For this review, take the finished solid that the model builds, in its own axes (mm). Face numbers are marked on the shaded views. A direction names the side the tool comes from. Coordinates: 2 decimals unless noted, no trailing zeros. Loops run counter-clockwise (first coordinate to the right, second up) from the corner with the lowest first, then second, coordinate; pieces in that order, holes last.
Autodesk Inventor part; units mm, degrees
ref_plane "YZ Plane" through (0, 0, 0) normal (1, 0, 0) x (0, 1, 0)
ref_plane "XZ Plane" through (0, 0, 0) normal (0, 1, 0) x (-1, 0, 0)
ref_plane "XY Plane" through (0, 0, 0) normal (0, 0, 1) x (1, 0, 0)
sketch "Sketch1" plane through (0, 0, 0) normal (0, 1, 0) x (-1, 0, 0)
  line L0 (4, -2.4997) -> (79.711, -2.4997)
  line L1 (4, -103.4997) -> (4, -2.4997)
  line L2 (45, -103.4997) -> (4, -103.4997)
  line L3 (69.7122, -36.1325) -> (54.8327, -76.055)
  line L4 (54.8327, -76.055) -> (53.637, -79.4997)
  line L5 (53.637, -79.4997) -> (47.0364, -98.0359)
  line L6 (47.0364, -98.0359) -> (45, -103.4997)
  line L7 (79.711, -2.4997) -> (69.7122, -36.1325)
  line L8 (84.9819, 0) -> (0, 0)
  line L9 (75.6001, -30.2846) -> (84.9819, 0)
  line L10 (84.9819, 0) -> (75.6001, -30.2846)
  line L11 (70.9666, -42.7177) -> (65.5988, -57.1214)
  line L12 (61.2006, -68.9229) -> (56.067, -83.7178)
  line L13 (75.6001, -30.2846) -> (61.2006, -68.9229)
  line L14 (47.8016, -104.8767) -> (46.0595, -108.2232)
  line L15 (50.5948, -98.4014) -> (47.8016, -104.8767)
  line L16 (56.067, -83.7178) -> (50.5948, -98.4014)
  line L17 (0, -108.2232) -> (0, 0)
  line L18 (46.0595, -108.2232) -> (0, -108.2232)
  point P0 (0, 0)
  point P1 (-1, 0)
extrude "Extrusion1" add sketch "Sketch1" against normal blind 2.5 contours L0 L7 L3 L4 L5 L6 L2 L1 | L9 L13 L11 L12 L16 L15 L14 L18 L17 L8
extrude "Extrusion2" add sketch "Sketch1" along normal blind 111.5
properties part number "phoneBucketV2"
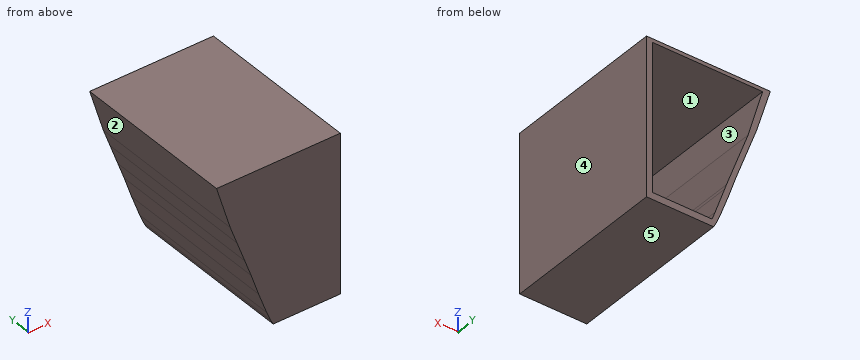
Q1. Machinability: for the marked faces 1 and 2, which of the approach directions +Z, -Z, +X, -X, +Y, -Y give a long, thin tool a straight path to every point of the face, cutting with its end or side? Answer none if there is none.
Q2. Consider section C-C (x = -22). State the section outline as (y, z) points.
Q3. Consider section B-B (z = -100). State the section outline as (x, y) points.
Q4. Consider section A-A (y = 89). State the section outline as (x, z) points (1 decimal).
Q5. Wall thickness on probe 1 along Z at (x, y) = (-43.5, 103); probe 2 along Y at (x, z) = (-58, -46); probe 3 along X at (y, z) = (67, -92): over which ranges is each line inside the solid? List them lowest first.
Q6. The part is to be moulded in two halves that separate along X. For the marked faces 3, 4 and 5, say which applies: +X half, -X half, draft (parallel to the pull), parting line (faces both ways), or undercut.
Q7. For pin 1 Ø3 at (x, z) = (-52.5, -16.5) entering from +Y; pin 2 Ø6 at (y, z) = (19, -37.5) entering from -X, all flat-tipped, find the tip position at first contact; note any pin that passes through.
Model answer:
1. face 1: +Y
1. face 2: -Z, -X, +Y, -Y
2. outline: (-2.5, -108.22) - (111.5, -108.22) - (111.5, -103.5) - (0, -103.5) - (0, -2.5) - (111.5, -2.5) - (111.5, 0) - (-2.5, 0) - close
3. outline: (-49.91, -2.5) - (0, -2.5) - (0, 111.5) - (-4, 111.5) - (-4, 0) - (-46.3, 0) - (-46.3, 111.5) - (-49.91, 111.5) - close
4. outline: (-85, 0) - (-75.6, -30.3) - (-71, -42.7) - (-65.6, -57.1) - (-61.2, -68.9) - (-56.1, -83.7) - (-50.6, -98.4) - (-47.8, -104.9) - (-46.1, -108.2) - (0, -108.2) - (0, 0) - close; hole (-79.7, -2.5) - (-69.7, -36.1) - (-54.8, -76.1) - (-53.6, -79.5) - (-47, -98) - (-45, -103.5) - (-4, -103.5) - (-4, -2.5) - close
5. probe 1: z = -108.22 to -103.5, -2.5 to 0
5. probe 2: y = -2.5 to 0
5. probe 3: x = -52.98 to -49.19, -4 to 0
6. face 3: undercut
6. face 4: +X half
6. face 5: draft
7. pin 1: stops at y = 0
7. pin 2: stops at x = -74.03
